Part model, mm, in its own coordinate system. A direction names the side the tool comes from. Round coordinates to 2 decimals unless told otherwise and drop trailing zeros. Write each loop counter-clockwise with the first axis right and the second up, starting at its lowest first coordinate (ties: lowest second). Pieces come first, ordered by that corner, then holes.
```python
from build123d import *

# Parameters (mm, degrees)
SKETCH_1_W          = 80
SKETCH_1_H          = 20
EXTRUDE_1_DEPTH     = 4
SKETCH_2_W          = 20
SKETCH_2_H          = 20
EXTRUDE_2_DEPTH     = 10
SKETCH_3_R          = 2.1
CUT_EXTRUDE_1_DEPTH = 20
SKETCH_4_R          = 2
CUT_EXTRUDE_2_DEPTH = 20


with BuildPart() as part:
    # 草图1 → 凸台-拉伸1 (new body)
    with BuildSketch(Plane.XY):
        with Locations((40, 10)):
            Rectangle(SKETCH_1_W, SKETCH_1_H)
    extrude(amount=EXTRUDE_1_DEPTH)

    # 草图2 → 凸台-拉伸2 (add)
    with BuildSketch(Plane.XY.offset(4)):
        with Locations((10, 10)):
            Rectangle(SKETCH_2_W, SKETCH_2_H)
        with Locations((70, 10)):
            Rectangle(SKETCH_2_W, SKETCH_2_H)
    extrude(amount=EXTRUDE_2_DEPTH)

    # 草图3 → 切除-拉伸1 (cut)
    with BuildSketch(Plane.XY.offset(14)):
        with Locations((10, 10)):
            Circle(SKETCH_3_R)
        with Locations((70, 10)):
            Circle(SKETCH_3_R)
    extrude(amount=-CUT_EXTRUDE_1_DEPTH, mode=Mode.SUBTRACT)

    # 草图4 → 切除-拉伸2 (cut)
    with BuildSketch(Plane(origin=(0, 0, 0), x_dir=(-1, 0, 0), z_dir=(0, 0, -1))):
        with Locations((-40, 10)):
            Circle(SKETCH_4_R)
    extrude(amount=-CUT_EXTRUDE_2_DEPTH, mode=Mode.SUBTRACT)


solid = part.part
```
Q1. Cut at D-D on x = 40. Write the cut outline in (y, z), plus the area to 3 significant figures.
Values follow:
outline: (0, 0) - (8, 0) - (8, 4) - (0, 4) - close; (12, 0) - (20, 0) - (20, 4) - (12, 4) - close
area: 64.0 mm2
Q2. Wall check: L1, parallel to Y at x = 70, z = 5.25; L2, parallel to Y at x = 40, z = 0.95; L3, parallel to X at y = 13.25, z = 8.75. Give the ranges that are in metal, low to high.
Values follow:
L1: y = 0 to 7.9, 12.1 to 20
L2: y = 0 to 8, 12 to 20
L3: x = 0 to 20, 60 to 80
Q3. Cut at A-A on z = 10. Write the cut outline in (x, y).
Values follow:
outline: (0, 0) - (20, 0) - (20, 20) - (0, 20) - close; (60, 0) - (80, 0) - (80, 20) - (60, 20) - close; hole circle Ø4.2 at (10, 10); hole circle Ø4.2 at (70, 10)
Q4. Cut at C-C on x = 10. Write the cut outline in (y, z), plus the area to 3 significant figures.
Values follow:
outline: (0, 0) - (7.9, 0) - (7.9, 14) - (0, 14) - close; (12.1, 0) - (20, 0) - (20, 14) - (12.1, 14) - close
area: 221 mm2
Q5. Cut at B-B on y = 10. Write the cut outline in (x, z), plus the area to 3 significant figures.
Values follow:
outline: (0, 0) - (7.9, 0) - (7.9, 14) - (0, 14) - close; (12.1, 0) - (38, 0) - (38, 4) - (20, 4) - (20, 14) - (12.1, 14) - close; (42, 0) - (67.9, 0) - (67.9, 14) - (60, 14) - (60, 4) - (42, 4) - close; (72.1, 0) - (80, 0) - (80, 14) - (72.1, 14) - close
area: 586 mm2
Q6. Mould opens along Y. For faces 3 (the flat face through (0, 10, 7)), 4 (the cylindrical face through (7.9, 10.09, 7.1)), 5 (the flat face through (39.4, 0, 3.8)) say: +Y half, -Y half, draft (parallel to the pull), parting line (faces both ways), or undercut.
Values follow:
face 3: draft
face 4: undercut
face 5: -Y half
Q7. Which spindle directions (+Z, -Z, +X, -X, +Y, -Y) get a long thin tool onto all of the face, cutting with end or side? Do faces 1 (the flat face through (20, 10, 9)), 2 (the flat face through (39, 8, 0)). Say none if no direction does.
Values follow:
face 1: +Z, +Y, -Y
face 2: -Z, +X, -X, +Y, -Y
